```python
from build123d import *

# Parameters (mm, degrees)
EXTRUDE_1_DEPTH      = 55.815
EXTRUDE_1_DEPTH_BACK = 4.185
EXTRUDE_4_DEPTH      = 24
SKETCH_13_R          = 1.45
EXTRUDE_5_DEPTH      = 6
EXTRUDE_START        = 6
SKETCH_14_R          = 1.45
EXTRUDE_6_DEPTH      = 6
SKETCH_15_W          = 77
SKETCH_15_H          = 37.999949308
EXTRUDE_7_DEPTH      = 2
CUT_EXTRUDE_2_DEPTH  = 38
FILLET_2_R           = 3
FILLET_3_R           = 3
FILLET_4_R           = 3


with BuildPart() as part:
    # 草图1 → 凸台-拉伸1 (new, two sides: drawn at the far end of the back side and taken through both)
    with BuildSketch(Plane.XY.offset(-EXTRUDE_1_DEPTH_BACK)):
        Polygon((0, 1.5), (30, 1.5), (40, 1.5), (40, -1.5), (-40, -1.5), (-40, 1.5), align=None)
    extrude(amount=EXTRUDE_1_DEPTH + EXTRUDE_1_DEPTH_BACK)

    # 草图11 → 凸台-拉伸4 (add)
    with BuildSketch(Plane(origin=(0, 1.5, 0), x_dir=(1, 0, 0), z_dir=(0, 1, 0))):
        Polygon((36.5, -9.329285225), (-36.5, -9.329285225), (-36.5, -43.329234533), (36.5, -43.329234533), (38.5, -43.329234533), (38.5, -45.329234533), (-38.5, -45.329234533), (-38.5, -9.329285225), (-38.5, -7.329285225), (36.5, -7.329285225), (38.5, -7.329285225), (38.5, -9.329285225), align=None)
    extrude(amount=EXTRUDE_4_DEPTH)

    # 草图13 → 凸台-拉伸5 (add)
    with BuildSketch(Plane.XY.offset(55.815)):
        with Locations(Location((-38.55, 0, 0), (0, 0, 180))):
            Circle(SKETCH_13_R)
        with Locations(Location((38.55, 0, 0), (0, 0, 180))):
            Circle(SKETCH_13_R)
    extrude(amount=EXTRUDE_5_DEPTH)

    # 草图14 → 凸台-拉伸6 (add)
    with BuildSketch(Plane(origin=(0, 0, -4.185), x_dir=(-1, 0, 0), z_dir=(0, 0, -1)).offset(EXTRUDE_START)):
        with Locations((-38.55, 0)):
            Circle(SKETCH_14_R)
        with Locations((38.55, 0)):
            Circle(SKETCH_14_R)
    extrude(amount=-EXTRUDE_6_DEPTH)

    # 草图15 → 凸台-拉伸7 (add)
    with BuildSketch(Plane(origin=(0, 25.5, 0), x_dir=(1, 0, 0), z_dir=(0, 1, 0))):
        with Locations((0, -26.329259879)):
            Rectangle(SKETCH_15_W, SKETCH_15_H)
    extrude(amount=EXTRUDE_7_DEPTH)

    # 草图16 → 切除-拉伸2 (cut)
    with BuildSketch(Plane.XY.offset(45.329234533)):
        with BuildLine():
            Line((-18.734540656, 26.451398681), (-35.362355257, 20.836811932))
            ThreePointArc((-35.362355257, 20.836811932), (-37.12868865, 17.766202685), (-34.058079403, 15.999869293))
            Line((-34.058079403, 15.999869293), (-17.260126249, 21.671905422))
            ThreePointArc((-17.260126249, 21.671905422), (-15.664993145, 24.781150117), (-18.734540656, 26.451398681))
        make_face()
        with BuildLine():
            Line((-35.510009127, 10.232259834), (12.313007681, 26.380291484))
            ThreePointArc((12.313007681, 26.380291484), (15.481413648, 24.811469112), (13.912591276, 21.643063146))
            Line((13.912591276, 21.643063146), (-33.910425533, 5.495031496))
            ThreePointArc((-33.910425533, 5.495031496), (-37.078831499, 7.063853868), (-35.510009127, 10.232259834))
        make_face()
        with BuildLine():
            Line((-11.608912214, 7.748065143), (33.910425533, 23.118231136))
            ThreePointArc((33.910425533, 23.118231136), (37.078831499, 21.549408764), (35.510009127, 18.381002798))
            Line((35.510009127, 18.381002798), (-10.009328619, 3.010836806))
            ThreePointArc((-10.009328619, 3.010836806), (-13.177734585, 4.579659177), (-11.608912214, 7.748065143))
        make_face()
        with BuildLine():
            Line((18.964604183, 7.516895213), (33.910425533, 12.563536189))
            ThreePointArc((33.910425533, 12.563536189), (37.078831499, 10.994713817), (35.510009127, 7.826307851))
            Line((35.510009127, 7.826307851), (20.564187778, 2.779666876))
            ThreePointArc((20.564187778, 2.779666876), (17.395781811, 4.348489247), (18.964604183, 7.516895213))
        make_face()
    extrude(amount=-CUT_EXTRUDE_2_DEPTH, mode=Mode.SUBTRACT)

    # 圆角2
    fillet_2_edges = [part.edges().sort_by_distance(p)[0] for p in [
        (-38.5, 27.5, 26.329259879),
    ]]
    fillet(fillet_2_edges, radius=FILLET_2_R)

    # 圆角3
    # the kernel refuses this fillet: 3 mm, written as the material it takes off along each edge
    with BuildSketch(Plane(origin=(-38.5, 1.5, 7.329285225), x_dir=(1, 0, 0), z_dir=(0, 1, 0))) as fillet_3_piece_1:
        with BuildLine():
            CenterArc((FILLET_3_R, -FILLET_3_R), FILLET_3_R, 90, 90)
            Line((0, -FILLET_3_R), (0, 0))
            Line((0, 0), (FILLET_3_R, 0))
        make_face()
    extrude(amount=23, mode=Mode.SUBTRACT)
    with BuildSketch(Plane(origin=(-35.5, 24.5, 7.329285225), x_dir=(-1, 0, 0), z_dir=(0, -1, 0))) as fillet_3_piece_2:
        with BuildLine():
            CenterArc((3 - FILLET_3_R, -FILLET_3_R), FILLET_3_R, 0, 90)
            Line((3, -FILLET_3_R), (3, 0))
            Line((3, 0), (3 - FILLET_3_R, 0))
        make_face()
    revolve(axis=Axis((-35.5, 24.5, 7.329285225), (0, 0, -1)), revolution_arc=90, mode=Mode.SUBTRACT)
    with BuildSketch(Plane(origin=(46, 27.5, 7.329285225), x_dir=(0, -1, 0), z_dir=(-1, 0, 0))) as fillet_3_piece_3:
        with BuildLine():
            CenterArc((FILLET_3_R, FILLET_3_R), FILLET_3_R, 180, 90)
            Line((0, FILLET_3_R), (0, 0))
            Line((0, 0), (FILLET_3_R, 0))
        make_face()
    extrude(amount=81.5, mode=Mode.SUBTRACT)

    # 圆角4
    # the kernel refuses this fillet: 3 mm, written as the material it takes off along each edge
    with BuildSketch(Plane(origin=(-35.5, 27.5, 45.329234533), x_dir=(0, -1, 0), z_dir=(1, 0, 0))) as fillet_4_piece_1:
        with BuildLine():
            CenterArc((FILLET_4_R, FILLET_4_R), FILLET_4_R, 180, 90)
            Line((0, FILLET_4_R), (0, 0))
            Line((0, 0), (FILLET_4_R, 0))
        make_face()
    extrude(amount=81.5, mode=Mode.SUBTRACT)
    with BuildSketch(Plane(origin=(-38.5, 1.5, 45.329234533), x_dir=(1, 0, 0), z_dir=(0, 1, 0))) as fillet_4_piece_2:
        with BuildLine():
            CenterArc((FILLET_4_R, FILLET_4_R), FILLET_4_R, 180, 90)
            Line((0, FILLET_4_R), (0, 0))
            Line((0, 0), (FILLET_4_R, 0))
        make_face()
    extrude(amount=23, mode=Mode.SUBTRACT)
    with BuildSketch(Plane(origin=(-35.5, 24.5, 45.329234533), x_dir=(-1, 0, 0), z_dir=(0, -1, 0))) as fillet_4_piece_3:
        with BuildLine():
            CenterArc((3 - FILLET_4_R, FILLET_4_R), FILLET_4_R, 270, 90)
            Line((3, FILLET_4_R), (3, 0))
            Line((3, 0), (3 - FILLET_4_R, 0))
        make_face()
    revolve(axis=Axis((-35.5, 24.5, 45.329234533), (0, 0, -1)), revolution_arc=90, mode=Mode.SUBTRACT)


solid = part.part
```
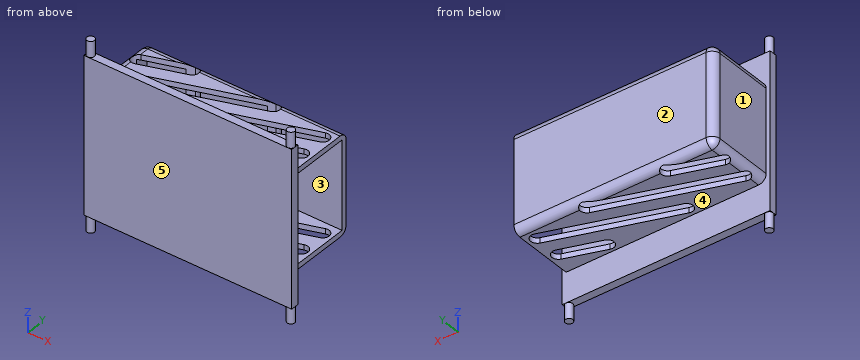
Geometry: final body of the model. Coordinates: model frame, mm. Face numbers are marked on the shaded views. A direction names the side the tool comes from. Round coordinates to 2 decimals unless told otherwise and drop trailing zeros. Order: outer loops, then holes, each group sorted by start corner. A loop starts at its lowest first (then second) coordinate and runs counter-clockwise, first axis right, second up. Notation, with made-up numbers: (-34.75, -3) - (2.25, -3) arc R24 ccw to (2.25, 32) - close; hole circle Ø7 at (14, 21.25). An arc over 180 degrees is marked (long way). Use CSV: the item, a comma, the result in double quotes. Start each with the question number.
Q1. Material intervals for line 1 along Y through (x, z) = (-9, 20); line 2 along Z through (x, y) = (-31, 2.25); line 3 along Y through (x, z) = (11, 1.5), sorted ascending. Write a range as from..to.
Q2. First-contact query: pin 1 (12.5 mm diameter, centred on x = -5.5, y = 19, fed in from +Z); pin 2 (7 mm diameter, centred on x = -14, y = 8.5, fed in from -Z); pin 3 (10 mm diameter, centred on x = 1, y = 4.5, fed in from +Z) (3 decimals); pin 4 (1.6 mm diameter, centred on x = -27, y = 22, fed in from -Z). Flat tips, straight axial feed; report the tip coordinate or a pass-through.
Q3. Section query A-A (z = 39). Return loops of the section in (x, y), and give its area (3 significant figures).
Q4. Access query for the marked faces 4 and 5. Directions: +Z, -Z, +X, -X, +Y, -Y. A direction counts if a zero-diameter tool reaches every point of the face in a straight line with its end or side. Return the directions, or none.
Q5. Section query B-B (x = -3). State how many separate pieces and enclosed holes the cut face has, and give its area (3 significant figures).
Q6. Mould query, pull axis Y, two halves, no side actions, for the marked faces 1, 2 and 3. Classes: +Y half, -Y half, draft (parallel to the pull), parting line (faces both ways), or undercut.
Result set:
1,line 1,"y = -1.5..1.5, 25.5..27.5"
1,line 2,"z = 7.33..9.33, 43.33..45.33"
1,line 3,"y = -1.5..1.5"
2,pin 1,"stops at z = 45.33"
2,pin 2,"stops at z = 7.33"
2,pin 3,"stops at z = 55.815"
2,pin 4,"passes through"
3,outline,"(-40, -1.5) - (40, -1.5) - (40, 1.5) - (-36.5, 1.5) - (-36.5, 6.12) arc R2.5 cw to (-36.5, 9.61) - (-36.5, 16.67) arc R2.5 cw to (-36.5, 20.17) - (-36.5, 25.5) - (-21.55, 25.5) - (-18.73, 26.45) arc R2.5 cw to (-16.02, 25.5) - (9.71, 25.5) - (12.31, 26.38) arc R2.5 cw to (15.12, 25.5) - (38.5, 25.5) - (38.5, 27.5) - (-35.5, 27.5) arc R3 ccw to (-38.5, 24.5) - (-38.5, 1.5) - (-40, 1.5) - close"
3,area,"430 mm2"
4,face 4,"-Z, +X, -X, +Y"
4,face 5,"+Z, -Z, +X, -X, -Y"
5,separate pieces,"4"
5,enclosed holes,"0"
5,area,"306 mm2"
6,face 1,"draft"
6,face 2,"+Y half"
6,face 3,"undercut"
